Model file for the job. Use its own axes, mm. A direction names the side the tool comes from. Give positions to 0.01 mm unless a question says otherwise; leave off trailing zeros. Write each loop counter-clockwise with the first axis right and the second up, starting at its lowest first coordinate (ties: lowest second). Pieces come first, ordered by that corner, then holes. Notation, with made-up numbers: (5, 25.25) - (37, 25.25) arc R16 cw to (37, 40.25) - close; hole circle Ø8 at (72, -9.75). An arc over 180 degrees is marked (long way). One line per item, written item: value. Start each with the question number.
(1) Drop flat-ended pins along their axis: P1, Ø0.8, axis at x = -3.5, z = 8, coming from the +Y side; P2, Ø3, axis at x = -5, z = 25.5, coming from the +Y side; P3, Ø1.2, axis at x = 2.5, y = 0, coming from the -Z side. Give the stop position or say it passes through.
(2) 3-axis set-ups, long thin cutter, end or side, ignore diameter. For faces 1 (the face through (3, -0.75, 5)), 2 (the face through (1, -2, 20)): which of +Z, -Z, +X, -X, +Y, -Y reach the whole face in a straight line?
(3) Probe L1, parallel to Y at x = 0, z = 26.25; L2, parallel to Z at x = 0.5, y = 3; L3, parallel to Y at x = 0, z = 17.5. List the from-to ranges inside material, lowest first.
(4) Cut at A-A, the plane y = 0. List the corners of the cut face in (x, z).
(5) Mould opens along X. For faces 3 (the face through (-1.7, 1.7, 9)), 4 (the face through (3, -1, 0)), 5 (the face through (-5.158, -3.955, 14.79)) say: pulls with the +X half, pulls with the -X half, needs draft (parallel to the pull), parting line crosses it, or undercut.
(6) Cut at D-D, the plane y = 3. List the corners of the cut face in (x, z), and give its area (3 significant figures).
(7) Cut at C-C, the plane z = 4.25. List the corners of the cut face in (x, y).
from build123d import *

# Parameters (mm, degrees)
SKETCH_R        = 6.5
SKETCH_R_2      = 2
PAD_DEPTH       = 30
SKETCH001_R     = 2.6
POCKET_DEPTH    = 10
SKETCH002_R     = 2.75
POCKET001_DEPTH = 9
SKETCH003_W     = 9
SKETCH003_H     = 1.5
SKETCH003_W_2   = 1.5
SKETCH003_H_2   = 9
POCKET002_DEPTH = 11


with BuildPart() as part:
    # Sketch → Pad (new body)
    with BuildSketch(Plane.XY):
        Circle(SKETCH_R)
        Circle(SKETCH_R_2, mode=Mode.SUBTRACT)
    extrude(amount=PAD_DEPTH)

    # Sketch001 → Pocket (cut)
    with BuildSketch(Plane.XY.offset(30)):
        Circle(SKETCH001_R)
    extrude(amount=-POCKET_DEPTH, mode=Mode.SUBTRACT)

    # Sketch002 → Pocket001 (cut)
    with BuildSketch(Plane(origin=(0, 0, 0), x_dir=(1, 0, 0), z_dir=(0, 0, -1))):
        Circle(SKETCH002_R)
    extrude(amount=-POCKET001_DEPTH, mode=Mode.SUBTRACT)

    # Sketch003 → Pocket002 (cut)
    with BuildSketch(Plane(origin=(0, 0, 0), x_dir=(1, 0, 0), z_dir=(0, 0, -1))):
        Rectangle(SKETCH003_W, SKETCH003_H)
        Rectangle(SKETCH003_W_2, SKETCH003_H_2)
    extrude(amount=-POCKET002_DEPTH, mode=Mode.SUBTRACT)


solid = part.part
Answers follow:
1. P1: stops at y = 5.71
1. P2: stops at y = 5.48
1. P3: stops at z = 11
2. face 1: -Z
2. face 2: +Z
3. L1: y = -6.5 to -2.6, 2.6 to 6.5
3. L2: z = 11 to 30
3. L3: y = -6.5 to -2, 2 to 6.5
4. outline: (-6.5, 0) - (-4.5, 0) - (-4.5, 11) - (-2, 11) - (-2, 20) - (-2.6, 20) - (-2.6, 30) - (-6.5, 30) - close; (2, 11) - (4.5, 11) - (4.5, 0) - (6.5, 0) - (6.5, 30) - (2.6, 30) - (2.6, 20) - (2, 20) - close
5. face 3: undercut
5. face 4: needs draft
5. face 5: parting line crosses it
6. outline: (-5.77, 0) - (-0.75, 0) - (-0.75, 11) - (0.75, 11) - (0.75, 0) - (5.77, 0) - (5.77, 30) - (-5.77, 30) - close
6. area: 329 mm²
7. outline: circle Ø13 at (0, 0); hole (-4.5, -0.75) - (-2.65, -0.75) arc R2.75 ccw to (-0.75, -2.65) - (-0.75, -4.5) - (0.75, -4.5) - (0.75, -2.65) arc R2.75 ccw to (2.65, -0.75) - (4.5, -0.75) - (4.5, 0.75) - (2.65, 0.75) arc R2.75 ccw to (0.75, 2.65) - (0.75, 4.5) - (-0.75, 4.5) - (-0.75, 2.65) arc R2.75 ccw to (-2.65, 0.75) - (-4.5, 0.75) - close
